Part model, mm, in its own coordinate system. Face numbers are marked on the shaded views. Round coordinates to 2 decimals unless told otherwise and drop trailing zeros. Loops run counter-clockwise (first coordinate to the right, second up) from the corner with the lowest first, then second, coordinate; pieces in that order, holes last.
from build123d import *

# Parameters (mm, degrees)
DODANIE_WYCI_GNI_CIE1_DEPTH = 17
SKORUPA2_T                  = -1.5
SZKIC5_R                    = 12.5
WYTNIJ_WYCI_GNI_CIE1_DEPTH  = 17


with BuildPart() as part:
    # Szkic1 → Dodanie-wyciągnięcie1 (new body)
    with BuildSketch(Plane.XY):
        Polygon((-9.604686356, 8), (-30.914686356, 8), (-28.684686356, -8), (-9.604686356, -8), align=None)
    extrude(amount=DODANIE_WYCI_GNI_CIE1_DEPTH)

    # Skorupa2
    skorupa2_openings = [part.faces().sort_by_distance(p)[0] for p in [
        (-19.144686356, -8, 8.5),
        (-20.259686356, 8, 8.5),
        (-9.604686356, 0, 8.5),
    ]]
    offset(amount=SKORUPA2_T, openings=skorupa2_openings, kind=Kind.INTERSECTION)

    # Szkic3 → Pogłębienie walcowe pod M2 Śrubę z łbem stożkowym ściętym1 (revolve, cut)
    with BuildSketch(Plane(origin=(-29.834614332, 0.250604313, 8.5), x_dir=(0.138040701, -0.990426557, 0), z_dir=(0, 0, 1))):
        Polygon((0, 0), (0, 10.721032743), (1.2, 10), (1.2, 1.6), (2.5, 1.6), (2.5, 0.025), (2.525, 0), align=None)
    revolve(axis=Axis((-36.123822969, -0.625954141, 8.5), (0.990426557, 0.138040701, 0)), mode=Mode.SUBTRACT)

    # Szkic5 → Wytnij-wyciągnięcie1 (cut)
    with BuildSketch(Plane(origin=(0, 8, 0), x_dir=(1, 0, 0), z_dir=(0, 1, 0))):
        with Locations((-0.439534966, -8.5)):
            Circle(SZKIC5_R)
    extrude(amount=-WYTNIJ_WYCI_GNI_CIE1_DEPTH, mode=Mode.SUBTRACT)


solid = part.part
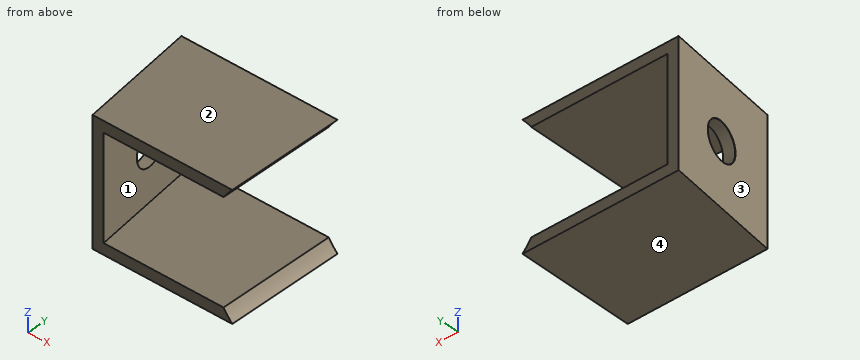
1) Slice it at A-A, the plane x = -16.25. Give the cut face in (y, z).
Values:
outline: (-8, 0) - (8, 0) - (8, 1.5) - (-8, 1.5) - close; (-8, 15.5) - (8, 15.5) - (8, 17) - (-8, 17) - close
2) Wall check: line 1 along Z through (x, y) = (-22.5, 7); line 2 along X through (y, z) = (6, 16); line 3 along X through (y, z) = (4.5, 16.25). Give the ranges that are in metal, low to high.
Values:
line 1: z = 0 to 1.5, 15.5 to 17
line 2: x = -30.64 to -10.44
line 3: x = -30.43 to -10.25
3) Slice it at C-C, the plane z = 4.5. Give the cut face in (x, y).
Values:
outline: (-30.91, 8) - (-28.68, -8) - (-27.17, -8) - (-29.4, 8) - close
4) Slice it at D-D, the plane y = -4.25. Give the cut face in (x, z).
Values:
outline: (-29.21, 0) - (-9.6, 0) arc R12.5 cw to (-10.8, 1.5) - (-27.69, 1.5) - (-27.69, 15.5) - (-10.8, 15.5) arc R12.5 cw to (-9.6, 17) - (-29.21, 17) - close
5) Drop flat-ended pins along their axis: pin 1 Ø2 at (x, z) = (-12.5, 3) entering from +Y; pin 2 Ø8 at (y, z) = (1, 4) entering from -X. Give the stop position or say it passes through.
Values:
pin 1: passes through
pin 2: stops at x = -30.5
6) Slice it at B-B, the plane y = 6.25. Give the cut face in (x, z).
Values:
outline: (-30.67, 0) - (-9.6, 0) arc R12.5 cw to (-10.8, 1.5) - (-29.16, 1.5) - (-29.16, 15.5) - (-10.8, 15.5) arc R12.5 cw to (-9.6, 17) - (-30.67, 17) - close
7) Mould opens along Z. For the marked faces 1, 2, 3 and 4 say: released by +Z, released by -Z, zero draft, split by the parting line, or undercut.
Values:
face 1: undercut
face 2: released by +Z
face 3: zero draft
face 4: released by -Z
